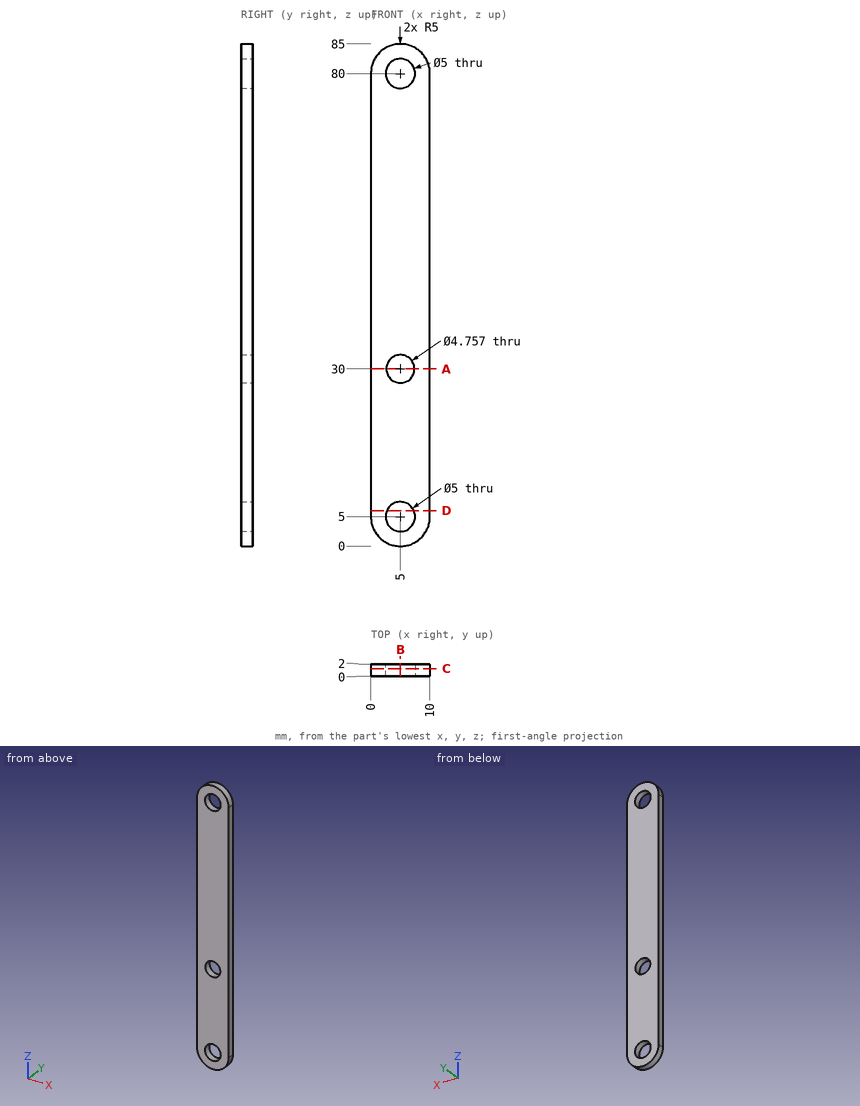
Geometry: see drawing. Coordinates: mm, zero at the bounding-box minimum. Give positions to 0.01 mm unless a question says otherwise; leave off trailing zeros. Order: outer loops, then holes, each group sorted by start corner. A loop starts at its lowest first (then second) coordinate and runs counter-clockwise, first axis right, second up.
1. Cut plane D-D (z = 6). Return loops of the section in (x, y), and give its area (3 significant figures).
Computed:
outline: (0, 0) - (2.71, 0) - (2.71, 2) - (0, 2) - close; (7.29, 0) - (10, 0) - (10, 2) - (7.29, 2) - close
area: 10.8 mm2
2. Pin query (flat end, axial travel): pin 1 Ø6 at (x, z) = (5, 30) entering from +Y; pin 2 Ø1 at (x, y) = (7.5, 1.5) entering from +Z. Return the tip coordinate at first contact, or that it passes through.
Computed:
pin 1: stops at y = 2
pin 2: stops at z = 84.58
3. Line query: probe 1 along Z at (x, y) = (5, 1.4); probe 2 along Z at (x, y) = (4, 0.5); probe 3 along X at (y, z) = (0.8, 80). Output: solid intervals per line, ascending.
Computed:
probe 1: z = 0 to 2.5, 7.5 to 27.62, 32.38 to 77.5, 82.5 to 85
probe 2: z = 0.1 to 2.71, 7.29 to 27.84, 32.16 to 77.71, 82.29 to 84.9
probe 3: x = 0 to 2.5, 7.5 to 10
4. Cut plane C-C (y = 1.25). Return loops of the section in (x, z).
Computed:
outline: (0, 5) arc R5 ccw to (10, 5) - (10, 80) arc R5 ccw to (0, 80) - close; hole circle Ø5 at (5, 5); hole circle Ø5 at (5, 80); hole circle Ø4.76 at (5, 30)
5. Cut plane A-A (z = 30). Return loops of the section in (x, y).
Computed:
outline: (0, 0) - (2.62, 0) - (2.62, 2) - (0, 2) - close; (7.38, 0) - (10, 0) - (10, 2) - (7.38, 2) - close
6. Cut plane B-B (x = 5). Return loops of the section in (y, z).
Computed:
outline: (0, 0) - (2, 0) - (2, 2.5) - (0, 2.5) - close; (0, 7.5) - (2, 7.5) - (2, 27.62) - (0, 27.62) - close; (0, 32.38) - (2, 32.38) - (2, 77.5) - (0, 77.5) - close; (0, 82.5) - (2, 82.5) - (2, 85) - (0, 85) - close
